Check sheet for the modelled part. Datum: model origin and axes. Units: mm. A direction names the side the tool comes from. Give positions to 0.01 mm unless a question says otherwise; leave off trailing zeros. Order: outer loops, then holes, each group sorted by start corner. A loop starts at its lowest first (then second) coordinate and runs counter-clockwise, first axis right, second up. Notation, with made-up numbers: (66, -35.5) - (124, -35.5) arc R14 ccw to (124, -24.5) - close; hole circle Ø2 at (-28, 46.5). An arc over 180 degrees is marked (long way). Answer in a Markdown table with one row per item.
from build123d import *

# Parameters (mm, degrees)
CROQUIS1_R              = 21.05
SALIENTE_EXTRUIR1_DEPTH = 13.25
REDONDEO1_R             = 1.5
CROQUIS2_R              = 4.45
CORTAR_EXTRUIR1_DEPTH   = 2
CROQUIS3_R              = 3.925
SALIENTE_EXTRUIR2_DEPTH = 13
CROQUIS4_R              = 5.908652193
SALIENTE_EXTRUIR3_DEPTH = 6.3
CROQUIS5_R              = 15.25
CROQUIS5_R_2            = 1.5
SALIENTE_EXTRUIR4_DEPTH = 2
CROQUIS6_R              = 2
SALIENTE_EXTRUIR5_DEPTH = 2.7
CROQUIS7_R              = 3
SALIENTE_EXTRUIR6_DEPTH = 1.2
CROQUIS8_W              = 3.5
CROQUIS8_H              = 3.439508105
SALIENTE_EXTRUIR7_DEPTH = 0.2
CROQUIS9_R              = 4.3
SALIENTE_EXTRUIR8_DEPTH = 7.4
CROQUIS10_R             = 6.65
SALIENTE_EXTRUIR9_DEPTH = 0.86


with BuildPart() as part:
    # Croquis1 → Saliente-Extruir1 (new body)
    with BuildSketch(Plane(origin=(0, 0, 0), x_dir=(1, 0, 0), z_dir=(0, 1, 0))):
        Circle(CROQUIS1_R)
    extrude(amount=SALIENTE_EXTRUIR1_DEPTH)

    # Redondeo1
    redondeo1_edges = [part.edges().sort_by_distance(p)[0] for p in [
        (-21.05, 13.25, 0),
    ]]
    fillet(redondeo1_edges, radius=REDONDEO1_R)

    # Croquis2 → Cortar-Extruir1 (cut)
    with BuildSketch(Plane(origin=(0, 13.25, 0), x_dir=(1, 0, 0), z_dir=(0, 1, 0))):
        with Locations((0.010957244, 12.691225968)):
            Circle(CROQUIS2_R)
        with Locations((10.996402716, 6.336123732)):
            Circle(CROQUIS2_R)
        with Locations((10.985445471, -6.355102236)):
            Circle(CROQUIS2_R)
        with Locations((-0.010957244, -12.691225968)):
            Circle(CROQUIS2_R)
        with Locations((-10.996402716, -6.336123732)):
            Circle(CROQUIS2_R)
        with Locations((-10.985445471, 6.355102236)):
            Circle(CROQUIS2_R)
    extrude(amount=-CORTAR_EXTRUIR1_DEPTH, mode=Mode.SUBTRACT)

    # Croquis3 → Saliente-Extruir2 (add)
    with BuildSketch(Plane(origin=(0, 13.25, 0), x_dir=(1, 0, 0), z_dir=(0, 1, 0))):
        Circle(CROQUIS3_R)
    extrude(amount=SALIENTE_EXTRUIR2_DEPTH)

    # Croquis4 → Saliente-Extruir3 (add)
    with BuildSketch(Plane.XZ):
        Circle(CROQUIS4_R)
    extrude(amount=SALIENTE_EXTRUIR3_DEPTH)

    # Croquis5 → Saliente-Extruir4 (add)
    with BuildSketch(Plane.XZ.offset(6.3)):
        Circle(CROQUIS5_R)
        with Locations((0, 12.5)):
            Circle(CROQUIS5_R_2, mode=Mode.SUBTRACT)
        with Locations((12.5, 0)):
            Circle(CROQUIS5_R_2, mode=Mode.SUBTRACT)
        with Locations((0, -12.5)):
            Circle(CROQUIS5_R_2, mode=Mode.SUBTRACT)
        with Locations((-12.5, 0)):
            Circle(CROQUIS5_R_2, mode=Mode.SUBTRACT)
    extrude(amount=SALIENTE_EXTRUIR4_DEPTH)

    # Croquis6 → Saliente-Extruir5 (add)
    with BuildSketch(Plane.XZ.offset(8.3)):
        Circle(CROQUIS6_R)
    extrude(amount=SALIENTE_EXTRUIR5_DEPTH)

    # Croquis7 → Saliente-Extruir6 (add)
    with BuildSketch(Plane.XZ.offset(8.3)):
        Circle(CROQUIS7_R)
    extrude(amount=SALIENTE_EXTRUIR6_DEPTH)

    # Croquis8 → Saliente-Extruir7 (add)
    with BuildSketch(Plane.XZ.offset(9.5)):
        with Locations((0, 1.730245948)):
            Rectangle(CROQUIS8_W, CROQUIS8_H)
    extrude(amount=SALIENTE_EXTRUIR7_DEPTH)

    # Croquis9 → Saliente-Extruir8 (add)
    with BuildSketch(Plane(origin=(0, 13.25, 0), x_dir=(1, 0, 0), z_dir=(0, 1, 0))):
        Circle(CROQUIS9_R)
    extrude(amount=SALIENTE_EXTRUIR8_DEPTH)

    # Croquis10 → Saliente-Extruir9 (add)
    with BuildSketch(Plane(origin=(0, 13.25, 0), x_dir=(1, 0, 0), z_dir=(0, 1, 0))):
        Circle(CROQUIS10_R)
    extrude(amount=SALIENTE_EXTRUIR9_DEPTH)


solid = part.part
(1) Access from +Z, -Z, +X, -X, +Y, -Y to the whole of each face (thin tool, end or side, straight path). Record for faces 4 (the flat face through (0, 11.25, -13)), 5 (the flat face through (0, 26.25, 0)), 6 (the cylindrical face through (0, -10, -2)), 7 (the flat face through (0, -6.3, -7)).
Geometry says:
| item | result |
|---|---|
| face 4 | +Y |
| face 5 | +Z, -Z, +X, -X, +Y |
| face 6 | -Y |
| face 7 | none |
(2) Thickness scan on L1, parallel to Y at x = -14.5, z = -1.5; L2, parallel to Y at x = 2.5, z = 15; L3, parallel to Z at x = 12.5, y = -7.45. Record the ranges inside material, lowest first.
Geometry says:
| item | result |
|---|---|
| L1 | -8.3 to -6.3, 0 to 13.25 |
| L2 | -8.3 to -6.3, 0 to 11.25 |
| L3 | -8.74 to -1.5, 1.5 to 8.74 |
(3) Gauge pin test, flat ends, axial feed: P1, Ø10, axis at x = -1.5, y = 6.5, coming from the -Z side; P2, Ø1.8, axis at x = 0, z = -12.5, coming from the -Y side; P3, Ø5, axis at x = -6, z = -4.5, coming from the +Y side. Record the tip position at first contact, or that the pin passes through.
Geometry says:
| item | result |
|---|---|
| P1 | z = -21.05 |
| P2 | y = 0 |
| P3 | y = 14.11 |
(4) Cross-section at A-A, the plane z = 0. Give the number of separate pieces and of enclosed holes in the cut face, then the cut area to 3 significant figures.
Geometry says:
| item | result |
|---|---|
| separate pieces | 3 |
| enclosed holes | 0 |
| area | 805 mm² |
(5) Cross-section at B-B, the plane y = -5. Record the cut outline in (x, z), then the cut area to 3 significant figures.
Geometry says:
| item | result |
|---|---|
| outline | circle Ø11.82 at (0, 0) |
| area | 110 mm² |
(6) Mould release check, pull along Z, two halves, no side actions. Record for faces 1 (the flat face through (0, -9.7, 3)), 2 (the cylindrical face through (-3, -9, 0)), 3 (the cylindrical face through (6.55, 12.26, -6.53)): pulls with the +Z half, pulls with the -Z half, needs draft (parallel to the pull), parting line crosses it, or undercut.
Geometry says:
| item | result |
|---|---|
| face 1 | needs draft |
| face 2 | parting line crosses it |
| face 3 | undercut |
